from build123d import *

# Parameters (mm, degrees)
SKETCH_W     = 42
SKETCH_H     = 42
PAD_DEPTH    = 40
CHAMFER_SIZE = 4
SKETCH001_R  = 11
PAD001_DEPTH = 2.5
SKETCH002_R  = 2.5
PAD002_DEPTH = 20
SKETCH003_R  = 1.5
POCKET_DEPTH = 7


with BuildPart() as part:
    # Sketch → Pad (new body)
    with BuildSketch(Plane.XY):
        Rectangle(SKETCH_W, SKETCH_H)
    extrude(amount=PAD_DEPTH)

    # Chamfer
    chamfer_edges = [part.edges().sort_by_distance(p)[0] for p in [
        (21, -21, 20),
        (-21, -21, 20),
        (-21, 21, 20),
        (21, 21, 20),
    ]]
    chamfer(chamfer_edges, length=CHAMFER_SIZE)

    # Sketch001 (on Face5 of Chamfer) → Pad001 (join)
    with BuildSketch(Plane.XY.offset(40)):
        Circle(SKETCH001_R)
    extrude(amount=PAD001_DEPTH)

    # Sketch002 (on Face12 of Pad001) → Pad002 (join)
    with BuildSketch(Plane.XY.offset(42.5)):
        Circle(SKETCH002_R)
    extrude(amount=PAD002_DEPTH)

    # Sketch003 (on Face5 of Pad002) → Pocket (cut)
    with BuildSketch(Plane.XY.offset(40)):
        with Locations((-15.5, 15.350468)):
            Circle(SKETCH003_R)
        with Locations((15.5, 15.350468)):
            Circle(SKETCH003_R)
        with Locations((15.5, -15.350468)):
            Circle(SKETCH003_R)
        with Locations((-15.5, -15.350468)):
            Circle(SKETCH003_R)
    extrude(amount=-POCKET_DEPTH, mode=Mode.SUBTRACT)


solid = part.part
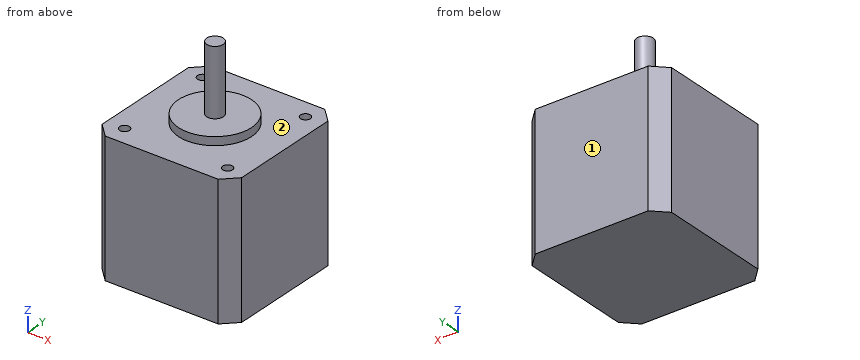
Design review of the part built by this model. Coordinates are the model's own, in mm. Face numbers are marked on the shaded views. A direction names the side the tool comes from. Give positions to 0.01 mm unless a question says otherwise; leave off trailing zeros. Order: outer loops, then holes, each group sorted by start corner. A loop starts at its lowest first (then second) coordinate and runs counter-clockwise, first axis right, second up.
1. Add section A-A, the plane y = 0. State the section outline as (x, z) points, then the cut area to 4 significant figures.
Solution:
outline: (-21, 0) - (21, 0) - (21, 40) - (11, 40) - (11, 42.5) - (2.5, 42.5) - (2.5, 62.5) - (-2.5, 62.5) - (-2.5, 42.5) - (-11, 42.5) - (-11, 40) - (-21, 40) - close
area: 1,835 mm2
2. Add section D-D, the plane z = 35. State the section outline as (x, y) points, then the cut area to 3 significant figures.
Solution:
outline: (-21, -17) - (-17, -21) - (17, -21) - (21, -17) - (21, 17) - (17, 21) - (-17, 21) - (-21, 17) - close; hole circle Ø3 at (-15.5, -15.35); hole circle Ø3 at (-15.5, 15.35); hole circle Ø3 at (15.5, -15.35); hole circle Ø3 at (15.5, 15.35)
area: 1,700 mm2
3. For pin 1 Ø2.5 at (x, y) = (16, 15) entering from +Z; pin 2 Ø1.5 at (x, y) = (-5.5, -0.5) entering from +Z; pin 3 Ø0.9 at (x, y) = (16, -15.5) entering from +Z, all flat-tipped, find the tip position at first contact; note any pin that passes through.
Solution:
pin 1: stops at z = 40
pin 2: stops at z = 42.5
pin 3: stops at z = 33
4. Add section C-C, the plane z = 17. State the section outline as (x, y) points.
Solution:
outline: (-21, -17) - (-17, -21) - (17, -21) - (21, -17) - (21, 17) - (17, 21) - (-17, 21) - (-21, 17) - close
5. To check wall thickness, follow L1, parallel to Y at x = -15.5, z = 37.25; L2, parallel to Y at x = -15, z = 35; L3, parallel to Z at x = 10, y = -1. State the ranges of each line that lie inside material, in increasing order.
Solution:
L1: y = -21 to -16.85, -13.85 to 13.85, 16.85 to 21
L2: y = -21 to -16.76, -13.94 to 13.94, 16.76 to 21
L3: z = 0 to 42.5
6. Tool access review of the marked faces 1 and 2: name each direction out of +Z, -Z, +X, -X, +Y, -Y from which nothing blocks a thin tool from reaching the whole face with its end or side.
Solution:
face 1: +Z, -Z, +X, -X, +Y
face 2: +Z
